Here's how the part is built. I have some questions about the finished solid (model axes, mm). A direction names the side the tool comes from. Coordinates: 2 decimals unless noted, no trailing zeros. Loops run counter-clockwise (first coordinate to the right, second up) from the corner with the lowest first, then second, coordinate; pieces in that order, holes last. Notation, with made-up numbers: (27.25, 85) - (75.25, 85) arc R4 cw to (75.25, 90) - close; hole circle Ø6 at (-35, 23). An arc over 180 degrees is marked (long way). Use a Markdown table: item, result.
```python
from build123d import *

# Parameters (mm, degrees)
F0_W     = 3.975
F0_H     = 13.5
F2_W     = 5
F2_H     = 10
F2_H_2   = 1.897511
F3_DEPTH = 25
F4_R     = 2.625
F5_DEPTH = 6
F6_R     = 2.625
F7_DEPTH = 6


with BuildPart() as f1:
    # F0 (on Top) → F1 (revolve)
    with BuildSketch(Plane.XY):
        Rectangle(F0_W, F0_H)
    revolve(axis=Axis((-1.9875, 0, 0), (0, -1, 0)))

    # F2 (on Right) → F3 (cut)
    with BuildSketch(Plane.YZ):
        with Locations((0, -8.2)):
            Rectangle(F2_W, F2_H)
        with Locations((0, 4.148756)):
            Rectangle(F2_W, F2_H_2)
    extrude(amount=-F3_DEPTH, mode=Mode.SUBTRACT)

    # F4 (on face) → F5 (cut)
    with BuildSketch(Plane.XZ.offset(6.75)):
        with Locations((-1.9875, 0)):
            Circle(F4_R)
    extrude(amount=-F5_DEPTH, mode=Mode.SUBTRACT)

    # F6 (on face) → F7 (cut)
    with BuildSketch(Plane(origin=(0, 6.75, 0), x_dir=(-1, 0, 0), z_dir=(0, 1, 0))):
        with Locations((1.9875, 0)):
            Circle(F6_R)
    extrude(amount=-F7_DEPTH, mode=Mode.SUBTRACT)


solid = f1.part
```
Q1. Will these pins go through, and if not, where does the flat tip stop? P1, Ø4, axis at x = -2.5, z = 0, coming from the -Y side; P2, Ø3, axis at y = 4, z = 2, coming from the -X side; P3, Ø2, axis at x = -2.5, y = 0, coming from the -Z side.
Check values:
| item | result |
|---|---|
| P1 | y = -0.75 |
| P2 | x = -5.93 |
| P3 | z = -3.2 |
Q2. I want a section at C-C, the plane x = -2.5. Write out the boundary of the cut face in (y, z).
Check values:
| item | result |
|---|---|
| outline | (-6.75, -3.94) - (-2.5, -3.94) - (-2.5, -3.2) - (2.5, -3.2) - (2.5, -3.94) - (6.75, -3.94) - (6.75, -2.57) - (0.75, -2.57) - (0.75, 2.57) - (6.75, 2.57) - (6.75, 3.94) - (2.5, 3.94) - (2.5, 3.2) - (-2.5, 3.2) - (-2.5, 3.94) - (-6.75, 3.94) - (-6.75, 2.57) - (-0.75, 2.57) - (-0.75, -2.57) - (-6.75, -2.57) - close |
Q3. I want a section at B-B, the plane z = -0.75. Write out the boundary of the cut face in (x, y).
Check values:
| item | result |
|---|---|
| outline | (-5.89, -6.75) - (-4.5, -6.75) - (-4.5, -0.75) - (0.53, -0.75) - (0.53, -6.75) - (1.92, -6.75) - (1.92, 6.75) - (0.53, 6.75) - (0.53, 0.75) - (-4.5, 0.75) - (-4.5, 6.75) - (-5.89, 6.75) - close |
Q4. Please list where these lines run through material, in increasing order: L1, parallel to X at y = -1.75, z = 1; L2, parallel to Y at x = -0.75, z = 1.75; L3, parallel to Z at x = 0.25, y = -1. Write a range as from..to.
Check values:
| item | result |
|---|---|
| L1 | -5.83..-4.41, 0.44..1.86 |
| L2 | -0.75..0.75 |
| L3 | -3.29..-1.37, 1.37..3.29 |
Q5. If we mould it in two halves opening along Y, with no side actions, what happens to faces 4 (the face through (-2, 0, -3.2)), 5 (the face through (-5, 6.75, -1)), 6 (the face through (-2, -0.75, 0))? For each: pulls with the +Y half, pulls with the -Y half, needs draft (parallel to the pull), parting line crosses it, or undercut.
Check values:
| item | result |
|---|---|
| face 4 | undercut |
| face 5 | pulls with the +Y half |
| face 6 | pulls with the -Y half |
Q6. Which directions (+Z, -Z, +X, -X, +Y, -Y) give clear straight access to the entire face, cutting with the end or side of a thin tool? Please do faces 1 (the face through (-2, 0.75, 0)), 2 (the face through (-3.9, -3.8, 1.8)), 3 (the face through (-2, 0, 3.2)).
Check values:
| item | result |
|---|---|
| face 1 | +Y |
| face 2 | -Y |
| face 3 | +Z, -X |
